Autodesk Inventor part; units mm, degrees
ref_plane "YZ Plane" through (0, 0, 0) normal (1, 0, 0) x (0, 1, 0)
ref_plane "XZ Plane" through (0, 0, 0) normal (0, 1, 0) x (-1, 0, 0)
ref_plane "XY Plane" through (0, 0, 0) normal (0, 0, 1) x (1, 0, 0)
sketch "스케치1" plane through (0, 0, 0) normal (0, 0, 1) x (1, 0, 0)
  circle A0 centre (0, 0) radius 2.7
  dimension "d0" = 5.4
extrude "돌출1" add sketch "스케치1" along normal blind 1.2
sketch "스케치2" plane through (0, 0, 1.2) normal (0, 0, 1) x (1, 0, 0)
  circle A0 centre (0, 0) radius 1.75
  dimension "d3" = 3.5
extrude "돌출2" add sketch "스케치2" along normal blind 4.8
hole "구멍1" at (-0.0349, 0.0291, 6) direction (0, 0, -1) diameter 2.459 depth 5 tip angle 118
properties part number "240621_나사"
Could you check a few things on this model? Use its own coordinates, in mm. A direction names the side the tool comes from. Coordinates: 2 decimals unless noted, no trailing zeros. Write each loop counter-clockwise with the first axis right and the second up, starting at its lowest first coordinate (ties: lowest second). Pieces come first, ordered by that corner, then holes. Notation, with made-up numbers: (47.25, 81.5) - (58.25, 81.5) arc R11 ccw to (58.25, 88.5) - close; hole circle Ø4 at (-5, 85). An arc over 180 degrees is marked (long way). Put each result on its own line as item: value. Start each with the question number.
Q1. I want a section at A-A on x = -1.45. Write out the boundary of the cut face in (y, z), plus the area to 3 significant figures.
Q2. Thinking about a two-plate mould opening in Y: for faces 1 (the flat face through (0, 0, 0)), 2 (the cylindrical face through (1.056, -0.538, 3.465)), 3 (the cylindrical face through (1.617, 0.67, 3.566)), which applies, pulls with the +Y half, pulls with the -Y half, needs draft (parallel to the pull), parting line crosses it, or undercut?
Q3. Please list where these lines run through material, in increasing order: L1, parallel to X at y = -0.05, z = 3.45; L2, parallel to Z at x = 0.45, y = 1.8; L3, parallel to Y at x = 0.45, z = 5.4.
Q4. I want a section at D-D on z = 0.5. Write out the boundary of the cut face in (x, y), plus the area to 3 significant figures.
Q5. Which directions (+Z, -Z, +X, -X, +Y, -Y) give clear straight access to the entire face, cutting with the end or side of a thin tool? Please do faces 4 (the cylindrical face through (-0.585, 2.636, 0.592)), 5 (the flat face through (0, -2, 1.2)).
Q6. I'm going to push a flat-ended pin straight in: P1, Ø3, axis at x = 1.5, z = 4.5, coming from the -Y side. Where does the tip first touch, or does it pass through?
Q7. I want a section at C-C on z = 5.6. Write out the boundary of the cut face in (x, y), plus the area to 3 significant figures.
Checks:
1. outline: (-2.28, 0) - (2.28, 0) - (2.28, 1.2) - (0.98, 1.2) - (0.98, 6) - (-0.98, 6) - (-0.98, 1.2) - (-2.28, 1.2) - close
1. area: 14.9 mm²
2. face 1: needs draft
2. face 2: undercut
2. face 3: parting line crosses it
3. L1: -1.75 to -1.26, 1.19 to 1.75
3. L2: 0 to 1.2
3. L3: -1.69 to -1.1, 1.16 to 1.69
4. outline: circle Ø5.4 at (0, 0); hole circle Ø0.79 at (-0.03, 0.03)
4. area: 22.4 mm²
5. face 4: +Z, -Z
5. face 5: +Z
6. P1: y = -1.75
7. outline: circle Ø3.5 at (0, 0); hole circle Ø2.46 at (-0.03, 0.03)
7. area: 4.87 mm²
